Verification items for the finished model (mm, model axes). A direction names the side the tool comes from. Give positions to 0.01 mm unless a question says otherwise; leave off trailing zeros. Loops run counter-clockwise (first coordinate to the right, second up) from the corner with the lowest first, then second, coordinate; pieces in that order, holes last. Notation, with made-up numbers: M 28,-19 L 74,-19 A17 cw 74,-7 Z; hole C 69,3.25 d9. An arc over 180 degrees is marked long. Use a Markdown table: item, result.
from build123d import *

# Parameters (mm, degrees)
F1_DEPTH   = 3.81
F2_W       = 8.128
F2_H       = 1.905
F1_FACE1_W = 20.6248
F1_FACE1_H = 3.81
F3_DEPTH   = 1.8542
F4_DEPTH   = 2.1844
F5_DEPTH   = 2.1844
F6_W       = 8.128
F6_H       = 2.1333807143
F7_DEPTH   = 6.096
F8_DEPTH   = 2.54
F9_DEPTH   = 2.54
F10_DEPTH  = 2.54
F11_DEPTH  = 6.096
F12_R      = 1.4742196791
F12_R_2    = 1.4703350309
F12_R_3    = 1.4763746717
F12_R_4    = 1.4703336231
F13_DEPTH  = 25.4
F16_DEPTH  = 2.0574
F18_DEPTH  = 1.27
F19_ANGLE  = -180


with BuildPart() as f1:
    # F0 (on Top) → F1 (new body)
    with BuildSketch(Plane.XY):
        Polygon((-10.3124, -9.2075), (10.3124, -9.2075), (10.3124, 9.2075), (4.064, 9.1750113802), (4.064, 3.0790113802), (-4.064, 3.0790113802), (-4.064, 9.1750113802), (-10.3124, 9.2075), align=None)
    extrude(amount=F1_DEPTH)

    # F2 (on face) + F1_face1 (on face) → F3 (join)
    with BuildSketch(Plane(origin=(0, 3.0790113802, 0), x_dir=(-1, 0, 0), z_dir=(0, 1, 0))):
        with Locations((0, 2.8575)):
            Rectangle(F2_W, F2_H)
    with BuildSketch(Plane(origin=(0, -9.2075, 1.905), x_dir=(1, 0, 0), z_dir=(0, -1, 0))):
        Rectangle(F1_FACE1_W, F1_FACE1_H)
    extrude(amount=-F3_DEPTH, dir=(0, 1, 0))

    # F4 (add): a face of the model
    f4_faces = [f1.faces().sort_by_distance(p)[0] for p in [
        (-10.3124, -0.9271, 1.905),
    ]]
    extrude(f4_faces, amount=F4_DEPTH)

    # F5 (add): a face of the model
    f5_faces = [f1.faces().sort_by_distance(p)[0] for p in [
        (10.3124, -0.9271, 1.905),
    ]]
    extrude(f5_faces, amount=F5_DEPTH)

    # F6 (on face) → F7 (join)
    with BuildSketch(Plane(origin=(0, 3.0790113802, 0), x_dir=(-1, 0, 0), z_dir=(0, 1, 0))):
        with Locations((0, 2.7433096429)):
            Rectangle(F6_W, F6_H)
    extrude(amount=F7_DEPTH)

    # F8 (add): a face of the model
    f8_faces = [f1.faces().sort_by_distance(p)[0] for p in [
        (-12.4968, -0.9271, 1.905),
    ]]
    extrude(f8_faces, amount=F8_DEPTH)

    # F9 (add): a face of the model
    f9_faces = [f1.faces().sort_by_distance(p)[0] for p in [
        (12.4968, -0.9271, 1.905),
    ]]
    extrude(f9_faces, amount=F9_DEPTH)

    # F10 (add): a face of the model
    f10_faces = [f1.faces().sort_by_distance(p)[0] for p in [
        (0, -11.0617, 1.905),
    ]]
    extrude(f10_faces, amount=F10_DEPTH)

    # F11 (cut): a face of the model
    f11_faces = [f1.faces().sort_by_distance(p)[0] for p in [
        (0, 3.0790113802, 0.8383096429),
    ]]
    extrude(f11_faces, amount=F11_DEPTH, mode=Mode.SUBTRACT)

    # F12 (on face) → F13 (cut)
    with BuildSketch(Plane.XY.offset(3.81)):
        with Locations((11.9888, -10.5537)):
            Circle(F12_R)
        with Locations((-11.9888, -10.5537)):
            Circle(F12_R_2)
        with Locations((11.9888, 6.1595)):
            Circle(F12_R_3)
        with Locations((-11.9888, 6.1595)):
            Circle(F12_R_4)
    extrude(amount=-F13_DEPTH, mode=Mode.SUBTRACT)


with BuildPart() as f14_1:
    # F14: copy of F1
    add(f1.part.moved(Location((0, -28.956, 0))))


with BuildPart() as f1_1:
    add(f1.part)

    # F16 (add): a face of the model
    f16_faces = [f1_1.faces().sort_by_distance(p)[0] for p in [
        (0, 3.0790113802, 0.8383096429),
    ]]
    extrude(f16_faces, amount=F16_DEPTH)

    # F17 (on face) → F18 (cut)
    with BuildSketch(Plane(origin=(0, 0, 0), x_dir=(1, 0, 0), z_dir=(0, 0, -1))):
        Polygon((-1.905, -5.1364113802), (1.905, -5.1364113802), (1.905, 1.340843155), (15.0368, 1.340843155), (15.0368, 4.1735726409), (-1.905, 4.1735726409), align=None)
    extrude(amount=-F18_DEPTH, mode=Mode.SUBTRACT)


with BuildPart() as f1_2:
    # F19: moved
    add(f1_1.part.rotate(Axis((15.0368, -8.8876363204, 0), (0, -1, 0)), F19_ANGLE))


solid = f1_2.part
(1) Cross-section at D-D on x = 43. Record the cut outline in (y, z).
Results below:
| item | result |
|---|---|
| outline | M -13.6,-3.81 L -11.69,-3.81 L -11.69,0 L -13.6,0 Z; M -9.42,-3.81 L 5.03,-3.81 L 5.03,0 L -9.42,0 Z; M 7.29,-3.81 L 9.21,-3.81 L 9.21,0 L 7.29,0 Z |
(2) Cross-section at B-B on z = -0.6. Record the cut outline in (x, y), then the cut area to 3 significant figures.
Results below:
| item | result |
|---|---|
| outline | M 15.04,-13.6 L 45.11,-13.6 L 45.11,9.21 L 40.39,9.21 L 34.14,9.18 L 34.14,5.14 L 31.98,5.14 L 31.98,-4.17 L 15.04,-4.17 Z; M 15.04,-1.34 L 28.17,-1.34 L 28.17,5.14 L 26.01,5.14 L 26.01,9.18 L 19.76,9.21 L 15.04,9.21 Z; hole C 18.08,-10.55 d2.95; hole C 18.08,6.16 d2.95; hole C 42.06,-10.55 d2.94; hole C 42.06,6.16 d2.94 |
| area | 553 mm^2 |
(3) Gauge pin test, flat ends, axial feed: P1, Ø1.7, axis at x = 29.5, z = -3, coming from the +Y side (3 decimals); P2, Ø1.2, axis at x = 29, y = 7.5, coming from the +Z side. Record the tip position at first contact, or that the pin passes through.
Results below:
| item | result |
|---|---|
| P1 | y = 9.175 |
| P2 | z = -1.68 |
(4) Cross-section at C-C on y = -2.75. Record the cut outline in (x, z), then the cut area to 3 significant figures.
Results below:
| item | result |
|---|---|
| outline | M 15.04,-3.81 L 45.11,-3.81 L 45.11,0 L 31.98,0 L 31.98,-1.27 L 15.04,-1.27 Z |
| area | 93.1 mm^2 |
(5) Material ranges on line 1 (Y direction, x = 18, z = -2.8); line 2 (Y direction, x = 18, z = -0.55); line 3 (X direction, y = 5, z = -1.4), recorded low to high.
Results below:
| item | result |
|---|---|
| line 1 | -13.6 to -12.03, -9.08 to 4.69, 7.63 to 9.21 |
| line 2 | -13.6 to -12.03, -9.08 to -4.17, -1.34 to 4.69, 7.63 to 9.21 |
| line 3 | 15.04 to 17.17, 19 to 41.16, 42.97 to 45.11 |
(6) Set-up check for faces 1 (the flat face through (23, -4.174, -1)), 2 (the flat face through (30, 9.175, -3)), 3 (the flat face through (30, 7, -1.677)): record each of +Z, -Z, +X, -X, +Y, -Y from which the full face is reachable in a straight line by a thin tool's end or side.
Results below:
| item | result |
|---|---|
| face 1 | +Z, -X |
| face 2 | +Z, -Z, +Y |
| face 3 | +Z, +Y |
(7) Cross-section at A-A on x = 29. Record the cut outline in (y, z), then the cut area to 3 significant figures.
Results below:
| item | result |
|---|---|
| outline | M -13.6,-3.81 L 9.18,-3.81 L 9.18,-1.68 L 5.14,-1.68 L 5.14,-1.27 L -4.17,-1.27 L -4.17,0 L -13.6,0 Z |
| area | 68.2 mm^2 |
(8) Draft check along X on faces 4 (the flat face through (31.979, 0, -1)), 5 (the flat face through (22, -1.341, -1)), 6 (the flat face through (45.11, -2, -2)). Enter one of: +X half, -X half, draft (parallel to the pull), parting line (faces both ways), or undercut.
Results below:
| item | result |
|---|---|
| face 4 | undercut |
| face 5 | draft |
| face 6 | +X half |
